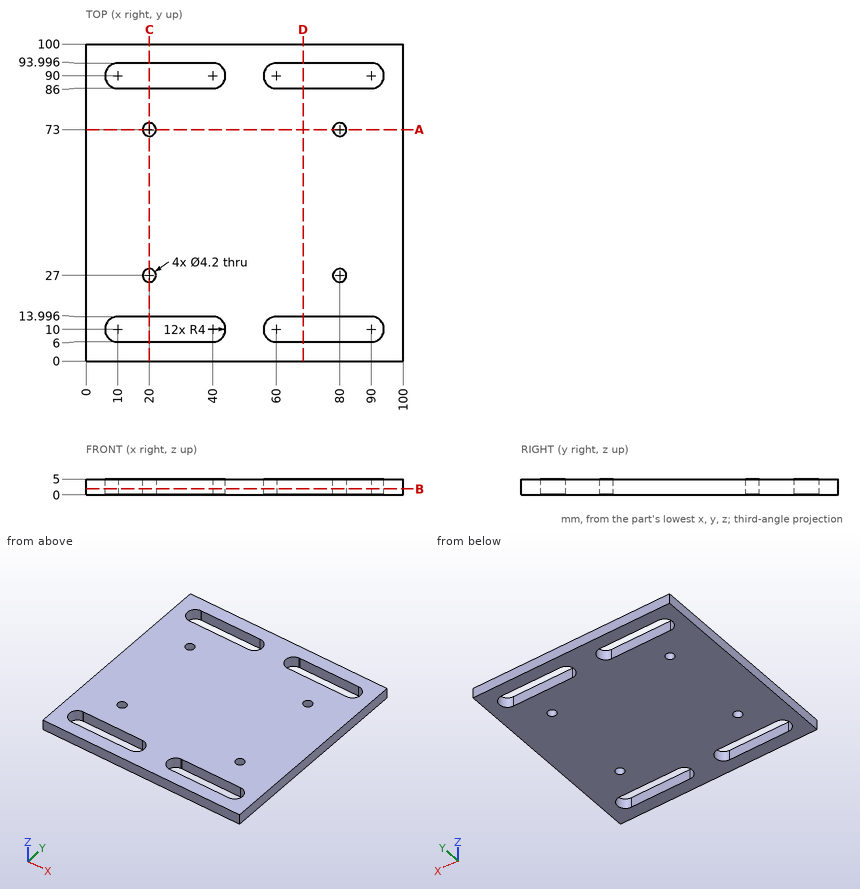
Here's the drawing with two shaded views (mm, measured from the low corner). I have some questions. Round coordinates to 2 decimals unless told otherwise and drop trailing zeros. Write each loop counter-clockwise with the first axis right and the second up, starting at its lowest first coordinate (ties: lowest second). Pieces come first, ordered by that corner, then holes. Notation, with made-up numbers: M 76,-27.5 L 84,-27.5 A25 cw 84,-5.5 Z; hole C 6,45.5 d11. An arc over 180 degrees is marked long. Answer in a Markdown table with one row per item. Add a question column.
Q1. If I drill on line 1 (Y direction, x = 24, z = 1.8); line 2 (Y direction, x = 20, z = 1.7); line 3 (X direction, y = 9, z = 2.6), over which ranges is the centre line in solid material (lowest first)? Write a range as from..to.
Q2. Imagine slicing it at A-A (y = 73). Please give me the cut outline in (x, z).
Q3. Imagine slicing it at B-B (z = 1.85). Give the number of separate pieces and of enclosed holes in the cut face, then the cut area to 3 significant figures.
Q4. Imagine slicing it at D-D (x = 68.5). Please give me the cut outline in (y, z).
Q5. Imagine slicing it at C-C (x = 20). Please give me the cut outline in (y, z).
Values:
| question | item | result |
|---|---|---|
| 1 | line 1 | 0..6, 14..86, 94..100 |
| 1 | line 2 | 0..6, 14..24.9, 29.1..70.9, 75.1..86, 94..100 |
| 1 | line 3 | 0..6.13, 43.87..56.13, 93.87..100 |
| 2 | outline | M 0,0 L 17.9,0 L 17.9,5 L 0,5 Z; M 22.1,0 L 77.9,0 L 77.9,5 L 22.1,5 Z; M 82.1,0 L 100,0 L 100,5 L 82.1,5 Z |
| 3 | separate pieces | 1 |
| 3 | enclosed holes | 8 |
| 3 | area | 8,780 mm^2 |
| 4 | outline | M 0,0 L 6,0 L 6,5 L 0,5 Z; M 14,0 L 86,0 L 86,5 L 14,5 Z; M 94,0 L 100,0 L 100,5 L 94,5 Z |
| 5 | outline | M 0,0 L 6,0 L 6,5 L 0,5 Z; M 14,0 L 24.9,0 L 24.9,5 L 14,5 Z; M 29.1,0 L 70.9,0 L 70.9,5 L 29.1,5 Z; M 75.1,0 L 86,0 L 86,5 L 75.1,5 Z; M 94,0 L 100,0 L 100,5 L 94,5 Z |
